```python
from build123d import *

# Parameters (mm, degrees)
SKETCH_1_W                 = 40
SKETCH_1_H                 = 10
SKETCH_1_H_2               = 15
EXTRUDE_1_DEPTH            = 6
SKETCH_3_R                 = 3
SKETCH_3_R_2               = 4
CUT_EXTRUDE_1_DEPTH        = 7
CUT_EXTRUDE_2_DEPTH        = 1
SKETCH_6_R                 = 2
EXTRUDE_2_DEPTH            = 5
SKETCH_7_R                 = 1.5
CUT_EXTRUDE_4_DEPTH        = 6
SKETCH_8_W                 = 10.1
SKETCH_8_H                 = 55
SKETCH_8_R                 = 1.5
CUT_EXTRUDE_5_DEPTH        = 1
SKETCH_9_R                 = 6
CUT_EXTRUDE_6_DEPTH        = 2
SKETCH_10_W                = 65
SKETCH_10_H                = 15
EXTRUDE_3_DEPTH            = 6
SKETCH_11_R                = 4
CUT_EXTRUDE_7_DEPTH        = 6
SKETCH_12_W                = 161.966486937
SKETCH_12_H                = 199.843871975
CUT_EXTRUDE_8_DEPTH        = 8
PATTERN_LINEAR_1_COUNT     = 3
PATTERN_LINEAR_1_PITCH     = 10
PATTERN_LINEAR_1_COL_COUNT = 3
PATTERN_LINEAR_1_COL_PITCH = 10
CHAMFER_1_SIZE             = 30
CHAMFER_1_SIZE2            = 50
FILLET_1_R                 = 10
EXTRUDE_4_DEPTH            = 5
FILLET_2_R                 = 10


with BuildPart() as part:
    # 草图1 → 凸台-拉伸1 (new body)
    with BuildSketch(Plane(origin=(0, 0, 0), x_dir=(1, 0, 0), z_dir=(0, 1, 0))):
        with Locations((20, -5)):
            Rectangle(SKETCH_1_W, SKETCH_1_H)
        with Locations((20, 7.5)):
            Rectangle(SKETCH_1_W, SKETCH_1_H_2)
        with Locations((20, -15)):
            Rectangle(SKETCH_1_W, SKETCH_1_H)
        Polygon((-20, 15), (-20, -20), (0, -20), (0, -10), (0, 0), (0, 15), align=None)
        Polygon((45, -20), (40, -20), (40, -10), (40, 0), (40, 15), (45, 15), align=None)
    extrude(amount=EXTRUDE_1_DEPTH)

    # 草图3 → 切除-拉伸1 (cut, through all)
    with BuildSketch(Plane(origin=(0, 6, 0), x_dir=(1, 0, 0), z_dir=(0, 1, 0))):
        with Locations((12.5, -6.5)):
            Circle(SKETCH_3_R)
        with Locations((-12.5, -6.5)):
            Circle(SKETCH_3_R_2)
    extrude(amount=-CUT_EXTRUDE_1_DEPTH, mode=Mode.SUBTRACT)

    # 草图4 → 切除-拉伸2 (cut)
    with BuildSketch(Plane(origin=(0, 6, 0), x_dir=(1, 0, 0), z_dir=(0, 1, 0))):
        with BuildLine():
            Line((6.5, -6.5), (9.5, -6.5))
            ThreePointArc((9.5, -6.5), (12.5, -3.5), (15.5, -6.5))
            ThreePointArc((15.5, -6.5), (14.621320344, -8.621320344), (12.5, -9.5))
            Line((12.5, -9.5), (12.5, -19))
            Line((12.5, -19), (21.5, -19))
            Line((21.5, -19), (21.5, 7))
            Line((21.5, 7), (6.5, 7))
            Line((6.5, 7), (6.5, -6.5))
        make_face()
        with BuildLine():
            ThreePointArc((12.5, -9.5), (10.378679656, -8.621320344), (9.5, -6.5))
            Line((9.5, -6.5), (6.5, -6.5))
            Line((6.5, -6.5), (6.5, -19))
            Line((6.5, -19), (12.5, -19))
            Line((12.5, -19), (12.5, -9.5))
        make_face()
    extrude(amount=-CUT_EXTRUDE_2_DEPTH, mode=Mode.SUBTRACT)

    # 草图6 → 凸台-拉伸2 (add)
    with BuildSketch(Plane.XY.offset(20)):
        Polygon((-20, 0), (12.5, 0), (45, 0), (45, 115), (-20, 115), align=None)
        with Locations((7.5, 81)):
            Circle(SKETCH_6_R, mode=Mode.SUBTRACT)
    extrude(amount=EXTRUDE_2_DEPTH)

    # 草图7 → 切除-拉伸4 (cut, through all)
    with BuildSketch(Plane(origin=(0, 0, 20), x_dir=(-1, 0, 0), z_dir=(0, 0, -1))):
        with Locations((-28, 87)):
            Circle(SKETCH_7_R)
    cut_extrude_4 = extrude(amount=-CUT_EXTRUDE_4_DEPTH, mode=Mode.SUBTRACT)

    # 草图8 → 切除-拉伸5 (cut)
    with BuildSketch(Plane(origin=(0, 0, 20), x_dir=(-1, 0, 0), z_dir=(0, 0, -1))):
        with Locations((-25.95, 87.5)):
            Rectangle(SKETCH_8_W, SKETCH_8_H)
        with Locations((-28, 87)):
            Circle(SKETCH_8_R, mode=Mode.SUBTRACT)
    extrude(amount=-CUT_EXTRUDE_5_DEPTH, mode=Mode.SUBTRACT)

    # 草图9 → 切除-拉伸6 (cut)
    with BuildSketch(Plane.XZ):
        with Locations((12.5, 6.5)):
            Circle(SKETCH_9_R)
    extrude(amount=-CUT_EXTRUDE_6_DEPTH, mode=Mode.SUBTRACT)

    # 草图10 → 凸台-拉伸3 (add)
    with BuildSketch(Plane.XZ):
        with Locations((12.5, -22.5)):
            Rectangle(SKETCH_10_W, SKETCH_10_H)
    extrude(amount=-EXTRUDE_3_DEPTH)

    # 草图11 → 切除-拉伸7 (cut)
    with BuildSketch(Plane(origin=(0, 6, 0), x_dir=(1, 0, 0), z_dir=(0, 1, 0))):
        with Locations((12.5, 18.5)):
            Circle(SKETCH_11_R)
    extrude(amount=-CUT_EXTRUDE_7_DEPTH, mode=Mode.SUBTRACT)

    # 草图12 → 切除-拉伸8 (cut)
    with BuildSketch(Plane(origin=(45, 0, 0), x_dir=(0, 0, -1), z_dir=(1, 0, 0))):
        with Locations((-40.373481837, 95.367627035)):
            Rectangle(SKETCH_12_W, SKETCH_12_H)
    extrude(amount=-CUT_EXTRUDE_8_DEPTH, mode=Mode.SUBTRACT)

    # 阵列(线性)1: 切除-拉伸4 ×3
    with Locations(*[(0, -i * PATTERN_LINEAR_1_PITCH, 0) for i in range(1, PATTERN_LINEAR_1_COUNT)]):
        add(cut_extrude_4, mode=Mode.SUBTRACT)

    # 阵列(线性)1 col: 切除-拉伸4 ×3
    with Locations(*[(0, i * PATTERN_LINEAR_1_COL_PITCH, 0) for i in range(1, PATTERN_LINEAR_1_COL_COUNT)]):
        add(cut_extrude_4, mode=Mode.SUBTRACT)

    # 倒角1
    chamfer_1_edges = [part.edges().sort_by_distance(p)[0] for p in [
        (-20, 115, 22.5),
    ]]
    chamfer_1_side = [part.faces().sort_by_distance(p)[0] for p in [
        (7.858875955, 115, 22.573481266),
    ]]
    chamfer(chamfer_1_edges, length=CHAMFER_1_SIZE, length2=CHAMFER_1_SIZE2, reference=chamfer_1_side[0])

    # 圆角1
    fillet_1_edges = [part.edges().sort_by_distance(p)[0] for p in [
        (-20, 65, 22.5),
        (10, 115, 22.5),
    ]]
    fillet(fillet_1_edges, radius=FILLET_1_R)

    # 草图13 → 凸台-拉伸4 (add)
    with BuildSketch(Plane(origin=(37, 0, 0), x_dir=(0, 0, -1), z_dir=(1, 0, 0))):
        Polygon((-20, 6), (0, 6), (-20, 46), align=None)
    extrude(amount=-EXTRUDE_4_DEPTH)

    # 圆角2
    fillet_2_edges = [part.edges().sort_by_distance(p)[0] for p in [
        (34.5, 46, 20),
        (34.5, 6, 0),
    ]]
    fillet(fillet_2_edges, radius=FILLET_2_R)


solid = part.part
```
Geometry check sheet. Reference: the model listing, model coordinates, mm. A direction names the side the tool comes from. Coordinates: 2 decimals unless noted, no trailing zeros. Order: outer loops, then holes, each group sorted by start corner. A loop starts at its lowest first (then second) coordinate and runs counter-clockwise, first axis right, second up.
Item 1: Section check D-D (x = 12.5). Enter the section's corners in (y, z), plus the area to 3 significant figures.
Item 2: Section check A-A (z = 6.5). Enter the section's corners in (x, y).
Item 3: Scan lines: line 1 along Y through (x, z) = (28, 21.9); line 2 along Z through (x, y) = (12.5, 1.4); line 3 along Z through (x, y) = (29.5, 78). Record each from-to range of solid material in increasing order.
Item 4: Section check C-C (x = -12.5). Enter the section's corners in (y, z), plus the area to 4 significant figures.
Item 5: Tool access check on faces 1 (the cylindrical face through (15.726, 0.986, 11.559)), 2 (the flat face through (16, 5, 6)), 3 (the flat face through (26, 88, 21)), 4 (the flat face through (8, 61, 20)). Record the directions out of +Z, -Z, +X, -X, +Y, -Y that give a thin tool (end or side, any length) a straight path to the whole face; none if there is none.
Item 6: Section check B-B (y = 97). Enter the section's corners in (x, z).
Item 7: Depth check by flat-ended pin: pin 1 (0.5 mm diameter, centred on x = 28, z = 20.5, fed in from +Y); pin 2 (9.5 mm diameter, centred on x = 13.5, z = 6.5, fed in from -Y); pin 3 (7 mm diameter, centred on x = 12.5, z = 6.5, fed in from +Y); pin 4 (3 mm diameter, centred on x = 27.5, z = -22.5, fed in from -Y). Enter the tip coordinate at first touch or a pass-through.
Item 8: Mould release check, pull along Y, two halves, no side actions. Record for faces 5 (the cylindrical face through (34.465, 7.534, -0.857)), 6 (the flat face through (15, 2, 4)), 7 (the cylindrical face through (28.195, 98.487, 22.972)), 8 (the flat face through (8, 58, 25)): released by +Y, released by -Y, zero draft, split by the parting line, or undercut.
Check sheet entries:
1. outline: (0, -30) - (6, -30) - (6, -22.5) - (0, -22.5) - close; (0, -14.5) - (6, -14.5) - (6, -7) - (5, -7) - (5, 3.5) - (2, 3.5) - (2, 0.5) - (0, 0.5) - close; (0, 12.5) - (2, 12.5) - (2, 9.5) - (5, 9.5) - (5, 19) - (6, 19) - (6, 20) - (114.49, 20) - (114.49, 25) - (0, 25) - close
1. area: 756 mm2
2. outline: (-20, 0) - (-16.5, 0) - (-16.5, 6) - (-20, 6) - close; (-8.5, 0) - (6.5, 0) - (6.5, 2) - (9.5, 2) - (9.5, 5) - (6.5, 5) - (6.5, 6) - (-8.5, 6) - close; (15.5, 2) - (18.5, 2) - (18.5, 0) - (37, 0) - (37, 19) - (32, 19) - (32, 6) - (21.5, 6) - (21.5, 5) - (15.5, 5) - close
3. line 1: y = 0 to 65.5, 68.5 to 75.5, 78.5 to 85.5, 88.5 to 95.5, 98.5 to 105.5, 108.5 to 115
3. line 2: z = -30 to -22.5, -14.5 to 0.5, 12.5 to 25
3. line 3: z = 21 to 25
4. outline: (0, -30) - (6, -30) - (6, 2.5) - (0, 2.5) - close; (0, 10.5) - (6, 10.5) - (6, 20) - (77.5, 20) - (77.5, 25) - (0, 25) - close
4. area: 639.5 mm2
5. face 1: -Y
5. face 2: +Y
5. face 3: -Z, +Y
5. face 4: -Z, -X, +Y
6. outline: (-0.8, 20) - (20.9, 20) - (20.9, 21) - (26.5, 21) - (26.5, 25) - (-0.8, 25) - close; (29.5, 21) - (31, 21) - (31, 20) - (37, 20) - (37, 25) - (29.5, 25) - close
7. pin 1: stops at y = 60
7. pin 2: stops at y = 2
7. pin 3: stops at y = 5
7. pin 4: stops at y = 0
8. face 5: released by +Y
8. face 6: released by -Y
8. face 7: undercut
8. face 8: zero draft
